Could you check a few things on this drawing? It's one solid part, dimensions in mm from its lowest x, y, z. A direction names the side the tool comes from. Coordinates: 2 decimals unless noted, no trailing zeros. Order: outer loops, then holes, each group sorted by start corner. A loop starts at its lowest first (then second) coordinate and runs counter-clockwise, first axis right, second up. Notation, with made-up numbers: (69, 49.5) - (122, 49.5) arc R17 ccw to (122, 71.5) - close; hole circle Ø10 at (57, 60). An arc over 180 degrees is marked (long way). Return JSON: item names as keys, results as strings. Group by question number.
1) Which directions (+Z, -Z, +X, -X, +Y, -Y) give clear straight access to the entire face, cutting with the end or side of a thin tool? Please do the marked faces 4, 5 and 6.
2) Imagine slicing it at B-B (x = 14.5). Write out the boundary of the cut face in (y, z), and give its area (3 significant figures).
3) Imagine slicing it at C-C (z = 5.25). Write out the boundary of the cut face in (x, y), and give its area (3 significant figures).
4) If we mould it in two halves opening along X, with no side actions, what happens to the marked faces 1, 2 and 3? For each: pulls with the +X half, pulls with the -X half, needs draft (parallel to the pull), parting line crosses it, or undercut.
5) Imagine slicing it at D-D (y = 6.4). Write out the boundary of the cut face in (x, z), and give its area (3 significant figures).
6) If I drill on line 1 along X through (y, z) = (2.5, 2.5); line 2 along X through (y, z) = (6.5, 1.25); line 3 along Y through (x, z) = (5, 4.5), over which ranges is the centre line in solid material (lowest first)?
7) For pin 1 Ø1.6 at (y, z) = (2.5, 3) entering from -X; pin 2 Ø1 at (y, z) = (1.5, 3) entering from +X, each with a flat end and sliding along its axis, tell me the tip position at first contact or that it passes through.
8) Imagine slicing it at A-A (y = 1.75). Write out the boundary of the cut face in (x, z), and give its area (3 significant figures).
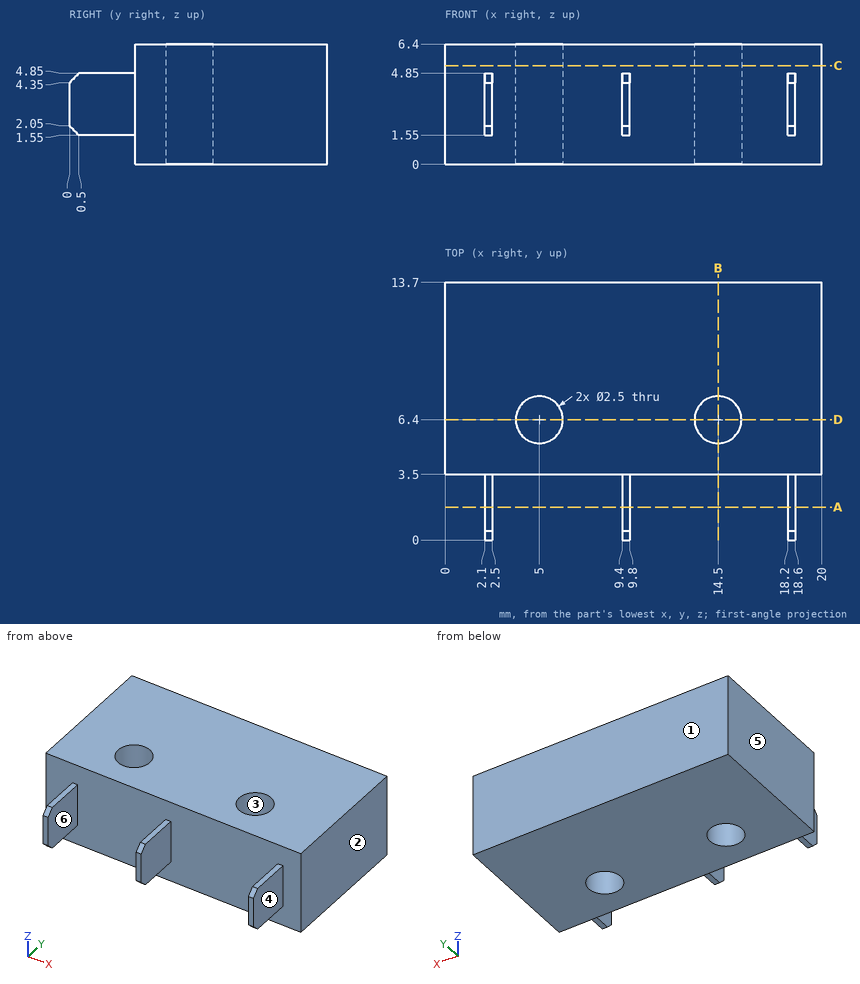
Calculated:
{
 "1": {"face 4": "+Z, -Z, +X, -Y", "face 5": "+Z, -Z, -X, +Y, -Y", "face 6": "+Z, -Z, -Y"},
 "2": {"outline": "(3.5, 0) - (5.15, 0) - (5.15, 6.4) - (3.5, 6.4) - close; (7.65, 0) - (13.7, 0) - (13.7, 6.4) - (7.65, 6.4) - close", "area": "49.3 mm2"},
 "3": {"outline": "(0, 3.5) - (20, 3.5) - (20, 13.7) - (0, 13.7) - close; hole circle Ø2.5 at (5, 6.4); hole circle Ø2.5 at (14.5, 6.4)", "area": "194 mm2"},
 "4": {"face 1": "needs draft", "face 2": "pulls with the +X half", "face 3": "undercut"},
 "5": {"outline": "(0, 0) - (3.75, 0) - (3.75, 6.4) - (0, 6.4) - close; (6.25, 0) - (13.25, 0) - (13.25, 6.4) - (6.25, 6.4) - close; (15.75, 0) - (20, 0) - (20, 6.4) - (15.75, 6.4) - close", "area": "96.0 mm2"},
 "6": {"line 1": "2.1 to 2.5, 9.4 to 9.8, 18.2 to 18.6", "line 2": "0 to 3.75, 6.25 to 13.25, 15.75 to 20", "line 3": "3.5 to 5.15, 7.65 to 13.7"},
 "7": {"pin 1": "x = 2.1", "pin 2": "x = 18.6"},
 "8": {"outline": "(2.1, 1.55) - (2.5, 1.55) - (2.5, 4.85) - (2.1, 4.85) - close; (9.4, 1.55) - (9.8, 1.55) - (9.8, 4.85) - (9.4, 4.85) - close; (18.2, 1.55) - (18.6, 1.55) - (18.6, 4.85) - (18.2, 4.85) - close", "area": "3.96 mm2"}
}
